Design review of the part built by this model. Coordinates are the model's own, in mm. A direction names the side the tool comes from. Give positions to 0.01 mm unless a question says otherwise; leave off trailing zeros. Write each loop counter-clockwise with the first axis right and the second up, starting at its lowest first coordinate (ties: lowest second). Pieces come first, ordered by that corner, then holes.
```python
from build123d import *

# Parameters (mm, degrees)
SKETCH2_W           = 81.6
SKETCH2_H           = 24
SKETCH2_W_2         = 77.6
SKETCH2_H_2         = 20
BOSS_EXTRUDE1_DEPTH = 8
SKETCH3_W           = 77.6
SKETCH3_H           = 20
BOSS_EXTRUDE2_DEPTH = 2
SKETCH4_R           = 2
SKETCH4_W           = 26.8
SKETCH4_H           = 19.5
SKETCH4_W_2         = 30.2
SKETCH4_H_2         = 14.3
CUT_EXTRUDE1_DEPTH  = 9
SKETCH6_W           = 30.2
SKETCH6_H           = 2.5
SKETCH6_W_2         = 1.7
SKETCH6_H_2         = 1.7
BOSS_EXTRUDE5_DEPTH = 5.2
SKETCH11_R          = 3
SKETCH11_R_2        = 2
BOSS_EXTRUDE6_DEPTH = 3.2
BOSS_EXTRUDE7_DEPTH = 2.7
SKETCH13_R          = 1.1
CUT_EXTRUDE2_DEPTH  = 4
CUT_EXTRUDE3_REACH  = 26
SKETCH15_W          = 10.1
SKETCH15_H          = 5.2
CHAMFER1_SIZE       = 1.5
SKETCH16_W          = 7
SKETCH16_H          = 12
CUT_EXTRUDE4_DEPTH  = 1.25


with BuildPart() as part:
    # Sketch2 → Boss-Extrude1 (new body)
    with BuildSketch(Plane(origin=(0, 0, 0), x_dir=(1, 0, 0), z_dir=(0, 1, 0))):
        Rectangle(SKETCH2_W, SKETCH2_H)
        Rectangle(SKETCH2_W_2, SKETCH2_H_2, mode=Mode.SUBTRACT)
    extrude(amount=BOSS_EXTRUDE1_DEPTH)

    # Sketch3 → Boss-Extrude2 (add)
    with BuildSketch(Plane(origin=(0, 0, 0), x_dir=(1, 0, 0), z_dir=(0, 1, 0))):
        Rectangle(SKETCH3_W, SKETCH3_H)
    extrude(amount=BOSS_EXTRUDE2_DEPTH)

    # Sketch4 → Cut-Extrude1 (cut, through all)
    with BuildSketch(Plane(origin=(0, 8, 0), x_dir=(1, 0, 0), z_dir=(0, 1, 0))):
        with Locations((4.8, 0)):
            Circle(SKETCH4_R)
        with Locations((-22.25, 0)):
            Rectangle(SKETCH4_W, SKETCH4_H)
        with Locations((23.7, 0)):
            Rectangle(SKETCH4_W_2, SKETCH4_H_2)
    extrude(amount=-CUT_EXTRUDE1_DEPTH, mode=Mode.SUBTRACT)

    # Sketch6 → Boss-Extrude5 (add)
    with BuildSketch(Plane(origin=(0, 2, 0), x_dir=(-1, 0, 0), z_dir=(0, 1, 0))):
        with Locations((-23.7, 8.75)):
            Rectangle(SKETCH6_W, SKETCH6_H)
        with Locations((-23.7, -8.75)):
            Rectangle(SKETCH6_W, SKETCH6_H)
        with Locations((37.95, 9.15)):
            Rectangle(SKETCH6_W_2, SKETCH6_H_2)
        with Locations((37.95, -9.15)):
            Rectangle(SKETCH6_W_2, SKETCH6_H_2)
    extrude(amount=BOSS_EXTRUDE5_DEPTH)

    # Sketch11 → Boss-Extrude6 (add)
    with BuildSketch(Plane(origin=(0, 2, 0), x_dir=(1, 0, 0), z_dir=(0, 1, 0))):
        with Locations((4.8, 0)):
            Circle(SKETCH11_R)
        with Locations((4.8, 0)):
            Circle(SKETCH11_R_2, mode=Mode.SUBTRACT)
    extrude(amount=BOSS_EXTRUDE6_DEPTH)

    # Sketch8 → Boss-Extrude7 (add)
    with BuildSketch(Plane(origin=(0, 2, 0), x_dir=(1, 0, 0), z_dir=(0, 1, 0))):
        with BuildLine():
            Line((-8.85, -9.75), (-8.85, -5.087533784))
            ThreePointArc((-8.85, -5.087533784), (-6.508058909, -5.323344034), (-5.4, -7.4))
            Line((-5.4, -7.4), (-5.4, -10))
            Line((-5.4, -10), (-8.85, -10))
            Line((-8.85, -10), (-8.85, -9.75))
        make_face()
        with BuildLine():
            Line((-5.4, 10), (-8.85, 10))
            Line((-8.85, 10), (-8.85, 9.75))
            Line((-8.85, 9.75), (-8.85, 5.287533784))
            ThreePointArc((-8.85, 5.287533784), (-6.508058909, 5.523344034), (-5.4, 7.6))
            Line((-5.4, 7.6), (-5.4, 10))
        make_face()
    extrude(amount=BOSS_EXTRUDE7_DEPTH)

    # Sketch13 → Cut-Extrude2 (cut)
    with BuildSketch(Plane(origin=(0, 4.7, 0), x_dir=(1, 0, 0), z_dir=(0, 1, 0))):
        with Locations((-7.9, 7.6)):
            Circle(SKETCH13_R)
        with Locations((-7.9, -7.4)):
            Circle(SKETCH13_R)
    extrude(amount=-CUT_EXTRUDE2_DEPTH, mode=Mode.SUBTRACT)

    # Sketch15 → Cut-Extrude3 (cut, up to next)
    with BuildSketch(Plane(origin=(0, 0, -12), x_dir=(-1, 0, 0), z_dir=(0, 0, -1)), mode=Mode.PRIVATE) as cut_extrude3_sk1:
        with Locations((26.35, 2.6)):
            Rectangle(SKETCH15_W, SKETCH15_H)
    cut_extrude3_tool1 = extrude(cut_extrude3_sk1.sketch, amount=-CUT_EXTRUDE3_REACH, mode=Mode.PRIVATE) & part.part
    add(cut_extrude3_tool1.solids().sort_by_distance((-26.35, 2.6, -12))[0], mode=Mode.SUBTRACT)

    # Chamfer1
    chamfer1_edges = [part.edges().sort_by_distance(p)[0] for p in [
        (-21.3, 2.6, -12),
        (-31.4, 2.6, -12),
        (-26.35, 5.2, -12),
    ]]
    chamfer(chamfer1_edges, length=CHAMFER1_SIZE)

    # Sketch16 → Cut-Extrude4 (cut)
    with BuildSketch(Plane(origin=(0, 2, 0), x_dir=(1, 0, 0), z_dir=(0, 1, 0))):
        with Locations((-1.7, 0)):
            Rectangle(SKETCH16_W, SKETCH16_H)
    extrude(amount=-CUT_EXTRUDE4_DEPTH, mode=Mode.SUBTRACT)


solid = part.part
```
(1) Clearance check with flat-ended pins moving along their axes: P1, Ø2, axis at x = 8.5, z = -2.5, coming from the -Y side; P2, Ø2.5, axis at x = -8, z = -7.5, coming from the +Y side; P3, Ø10, axis at x = 7, z = -1, coming from the +Y side; P4, Ø2, axis at x = -0.5, z = -0.5, coming from the +Y side. State where each tip first meets the part, or that it passes through.
Resolved:
P1: stops at y = 0
P2: stops at y = 4.7
P3: stops at y = 5.2
P4: stops at y = 0.75
(2) Consider section B-B, the plane x = -3. Give the boundary of the cut face in (y, z), then the cut area to 3 significant figures.
Resolved:
outline: (0, -12) - (8, -12) - (8, -10) - (2, -10) - (2, -6) - (0.75, -6) - (0.75, 6) - (2, 6) - (2, 10) - (8, 10) - (8, 12) - (0, 12) - close
area: 57.0 mm2
(3) Consider section D-D, the plane x = -16. Give the boundary of the cut face in (y, z).
Resolved:
outline: (0, -12) - (8, -12) - (8, -10) - (2, -10) - (2, -9.75) - (0, -9.75) - close; (0, 9.75) - (2, 9.75) - (2, 10) - (8, 10) - (8, 12) - (0, 12) - close
(4) Consider section A-A, the plane x = 12. Give the boundary of the cut face in (y, z).
Resolved:
outline: (0, -12) - (8, -12) - (8, -10) - (7.2, -10) - (7.2, -7.5) - (2, -7.5) - (2, -7.15) - (0, -7.15) - close; (0, 7.15) - (2, 7.15) - (2, 7.5) - (7.2, 7.5) - (7.2, 10) - (8, 10) - (8, 12) - (0, 12) - close
(5) Mouldability with a two-part tool opening along Z and no side actions: class faces 4 (the face through (-1, 4, 12)), 5 (the face through (-1, 4, -12)), 6 (the face through (40.8, 4, 0)), 7 (the face through (-2, 0.75, 0)) as pulls with the +Z half, pulls with the -Z half, needs draft (parallel to the pull), parting line crosses it, or undercut.
Resolved:
face 4: pulls with the +Z half
face 5: pulls with the -Z half
face 6: needs draft
face 7: undercut
(6) To check wall thickness, follow L1, parallel to X at y = 3.9, z = 0; L2, parallel to X at y = 0.5, z = 6.25; L3, parallel to X at y = 1, z = 4.5. State the ranges of each line that lie inside material, in increasing order.
Resolved:
L1: x = -40.8 to -38.8, 1.8 to 2.8, 6.8 to 7.8, 38.8 to 40.8
L2: x = -40.8 to -35.65, -8.85 to 8.6, 38.8 to 40.8
L3: x = -40.8 to -35.65, -8.85 to -5.2, 1.8 to 8.6, 38.8 to 40.8
(7) Tool access review of faces 1 (the face through (-38.8, 5, 0)), 2 (the face through (-34, 1, -9.75)), 3 (the face through (-40.8, 4, 0)): name each direction out of +Z, -Z, +X, -X, +Y, -Y from which nothing blocks a thin tool from reaching the whole face with its end or side.
Resolved:
face 1: +Y
face 2: +Y, -Y
face 3: +Z, -Z, -X, +Y, -Y
(8) Consider section C-C, the plane y = 4. Give the number of separate pieces and of enclosed holes in the cut face, then the cut area to 3 significant figures.
Resolved:
separate pieces: 2
enclosed holes: 1
area: 581 mm2
